Input: part model. Units: mm. Frame: model coordinates. Coordinates: 2 decimals unless noted, no trailing zeros. Loops run counter-clockwise (first coordinate to the right, second up) from the corner with the lowest first, then second, coordinate; pieces in that order, holes last. Notation, with made-up numbers: (30.25, 53) - (46.25, 53) arc R29 ccw to (46.25, 85) - close; hole circle Ø7 at (43, -18.75). An arc over 180 degrees is marked (long way). Use one line per item in the form item = value.
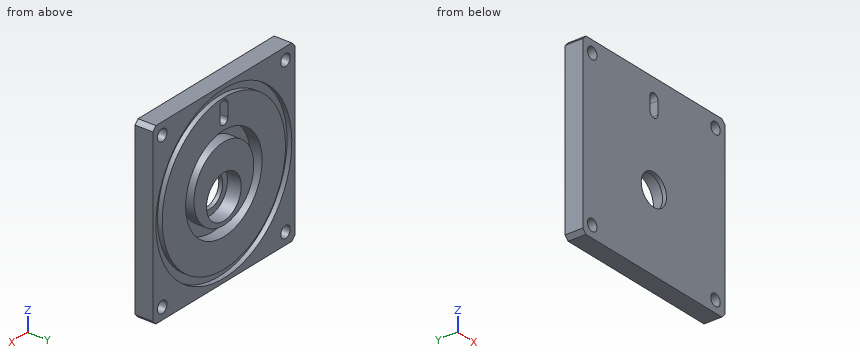
from build123d import *

# Parameters (mm, degrees)
SKETCH_1_W          = 45
SKETCH_1_H          = 45
EXTRUDE_1_DEPTH     = 4.5
SKETCH_2_R          = 5.5
CUT_EXTRUDE_1_DEPTH = 3.5
SKETCH_3_R          = 4
CUT_EXTRUDE_2_DEPTH = 33.011716605
SKETCH_4_R          = 12.1
SKETCH_4_R_2        = 9.45
CUT_EXTRUDE_3_DEPTH = 3
SKETCH_5_R          = 21.5
SKETCH_5_R_2        = 19.5
CUT_EXTRUDE_4_DEPTH = 1.2
CUT_EXTRUDE_5_DEPTH = 33.136427928
SKETCH_8_R          = 1.5
CUT_EXTRUDE_6_DEPTH = 33.136427928
CHAMFER_1_SIZE      = 1


with BuildPart() as part:
    # 草图1 → 凸台-拉伸1 (new body)
    with BuildSketch(Plane(origin=(0, 0, 0), x_dir=(1, 0, 0), z_dir=(0, 1, 0))):
        Rectangle(SKETCH_1_W, SKETCH_1_H)
    extrude(amount=EXTRUDE_1_DEPTH)

    # 草图2 → 切除-拉伸1 (cut)
    with BuildSketch(Plane(origin=(0, 4.5, 0), x_dir=(1, 0, 0), z_dir=(0, 1, 0))):
        with Locations(Location((0, 3, 0), (0, 0, 270))):
            Circle(SKETCH_2_R)
    extrude(amount=-CUT_EXTRUDE_1_DEPTH, mode=Mode.SUBTRACT)

    # 草图3 → 切除-拉伸2 (cut, through all)
    with BuildSketch(Plane(origin=(0, 1, 0), x_dir=(1, 0, 0), z_dir=(0, 1, 0))):
        with Locations(Location((0, 3, 0), (0, 0, 270))):
            Circle(SKETCH_3_R)
    extrude(amount=-CUT_EXTRUDE_2_DEPTH, mode=Mode.SUBTRACT)

    # 草图4 → 切除-拉伸3 (cut)
    with BuildSketch(Plane(origin=(0, 4.5, 0), x_dir=(1, 0, 0), z_dir=(0, 1, 0))):
        with Locations(Location((0, 0, 0), (0, 0, 270))):
            Circle(SKETCH_4_R)
        with Locations(Location((0, 0, 0), (0, 0, 270))):
            Circle(SKETCH_4_R_2, mode=Mode.SUBTRACT)
    extrude(amount=-CUT_EXTRUDE_3_DEPTH, mode=Mode.SUBTRACT)

    # 草图5 → 切除-拉伸4 (cut)
    with BuildSketch(Plane(origin=(0, 4.5, 0), x_dir=(1, 0, 0), z_dir=(0, 1, 0))):
        with Locations(Location((0, 0, 0), (0, 0, 270))):
            Circle(SKETCH_5_R)
        with Locations(Location((0, 0, 0), (0, 0, 270))):
            Circle(SKETCH_5_R_2, mode=Mode.SUBTRACT)
    extrude(amount=-CUT_EXTRUDE_4_DEPTH, mode=Mode.SUBTRACT)

    # 草图6 → 切除-拉伸5 (cut, through all)
    with BuildSketch(Plane(origin=(0, 4.5, 0), x_dir=(1, 0, 0), z_dir=(0, 1, 0))):
        with BuildLine():
            Line((1.25, -14.5), (1.25, -17.75))
            ThreePointArc((1.25, -17.75), (0, -19), (-1.25, -17.75))
            Line((-1.25, -17.75), (-1.25, -14.5))
            ThreePointArc((-1.25, -14.5), (0, -13.25), (1.25, -14.5))
        make_face()
    extrude(amount=-CUT_EXTRUDE_5_DEPTH, mode=Mode.SUBTRACT)

    # 草图8 → 切除-拉伸6 (cut, through all)
    with BuildSketch(Plane.XZ):
        with Locations(Location((-19.5, 19.5, 0), (0, 0, 270))):
            Circle(SKETCH_8_R)
        with Locations(Location((19.5, 19.5, 0), (0, 0, 90))):
            Circle(SKETCH_8_R)
        with Locations(Location((19.5, -19.5, 0), (0, 0, 270))):
            Circle(SKETCH_8_R)
        with Locations(Location((-19.5, -19.5, 0), (0, 0, 90))):
            Circle(SKETCH_8_R)
    extrude(amount=-CUT_EXTRUDE_6_DEPTH, mode=Mode.SUBTRACT)

    # 倒角1
    chamfer_1_edges = [part.edges().sort_by_distance(p)[0] for p in [
        (22.5, 2.25, 22.5),
        (-22.5, 2.25, 22.5),
        (-22.5, 2.25, -22.5),
        (22.5, 2.25, -22.5),
    ]]
    chamfer(chamfer_1_edges, length=CHAMFER_1_SIZE)


solid = part.part
Q1. Cut plane B-B, the plane z = -6. Return loops of the section in (x, y).
Check values:
outline = (-22.5, 0) - (-2.65, 0) - (-2.65, 1) - (-4.61, 1) - (-4.61, 4.5) - (-7.3, 4.5) - (-7.3, 1.5) - (-10.51, 1.5) - (-10.51, 4.5) - (-18.55, 4.5) - (-18.55, 3.3) - (-20.65, 3.3) - (-20.65, 4.5) - (-22.5, 4.5) - close; (2.65, 0) - (22.5, 0) - (22.5, 4.5) - (20.65, 4.5) - (20.65, 3.3) - (18.55, 3.3) - (18.55, 4.5) - (10.51, 4.5) - (10.51, 1.5) - (7.3, 1.5) - (7.3, 4.5) - (4.61, 4.5) - (4.61, 1) - (2.65, 1) - close
Q2. First-contact query: P1, Ø5.5, axis at x = 1.5, z = -1.5, coming from the +Y side. Flat tip, straight axial feed; report the tip coordinate or a pass-through.
Check values:
P1 = 1
Q3. Ray query, line 1 along X through (y, z) = (1.65, -19.5); line 2 along X through (y, z) = (2, 15); line 3 along Z through (x, y) = (-19, 2.95). Return the intervals inside material, ascending. Write a range as [from, to].
Check values:
line_1 = [-22.5, -21], [-18, 18], [21, 22.5]
line_2 = [-22.5, -1.25], [1.25, 22.5]
line_3 = [-22.5, -20.91], [-18.09, 18.09], [20.91, 22.5]
Q4. Cut plane A-A, the plane y = 2.2. Give the number of separate pieces and of enclosed holes in the cut face, then the cut area to 3 significant figures.
Check values:
separate_pieces = 2
enclosed_holes = 7
area = 1,710 mm²
Q5. Cut plane C-C, the plane x = -11. Return loops of the section in (y, z).
Check values:
outline = (0, -22.5) - (4.5, -22.5) - (4.5, -18.47) - (3.3, -18.47) - (3.3, -16.1) - (4.5, -16.1) - (4.5, -5.04) - (1.5, -5.04) - (1.5, 5.04) - (4.5, 5.04) - (4.5, 16.1) - (3.3, 16.1) - (3.3, 18.47) - (4.5, 18.47) - (4.5, 22.5) - (0, 22.5) - close
Q6. Cut plane D-D, the plane z = 5. Return loops of the section in (x, y).
Check values:
outline = (-22.5, 0) - (22.5, 0) - (22.5, 4.5) - (20.91, 4.5) - (20.91, 3.3) - (18.85, 3.3) - (18.85, 4.5) - (11.02, 4.5) - (11.02, 1.5) - (8.02, 1.5) - (8.02, 4.5) - (-8.02, 4.5) - (-8.02, 1.5) - (-11.02, 1.5) - (-11.02, 4.5) - (-18.85, 4.5) - (-18.85, 3.3) - (-20.91, 3.3) - (-20.91, 4.5) - (-22.5, 4.5) - close
